from build123d import *

# Parameters (mm, degrees)
SKETCH1_W           = 50
SKETCH1_H           = 50
BOSS_EXTRUDE1_DEPTH = 10
LOFT1_START         = -25
LOFT1_DEPTH         = 50
SKETCH4_R           = 1.6
CUT_EXTRUDE1_DEPTH  = 4
SKETCH6_R           = 1.6
CUT_EXTRUDE2_DEPTH  = 4
FILLET1_R           = 10
CUT_EXTRUDE4_DEPTH  = 1


# Read off the part's stored shape, not the designer's step: Loft1
with BuildPart() as part:
    # Sketch1 → Boss-Extrude1 (new body)
    with BuildSketch(Plane(origin=(0, 0, 0), x_dir=(1, 0, 0), z_dir=(0, 1, 0))):
        Rectangle(SKETCH1_W, SKETCH1_H)
    extrude(amount=BOSS_EXTRUDE1_DEPTH)

    # Loft1 outline → Loft1 (add)
    with BuildSketch(Plane.XY.offset(LOFT1_START)):
        Polygon((25, 0), (-25, 0), (24.904867452, -2.178893569), align=None)
    extrude(amount=LOFT1_DEPTH)

    # Sketch4 → Cut-Extrude1 (cut)
    with BuildSketch(Plane(origin=(-0.047566274, -1.089446784, 0), x_dir=(0.9990482215818578, -0.043619387365336104, 0), z_dir=(-0.043619387365336104, -0.9990482215818578, 0))):
        with Locations((20, 20)):
            Circle(SKETCH4_R)
        with Locations((20, -20)):
            Circle(SKETCH4_R)
        with Locations((-20, -20)):
            Circle(SKETCH4_R)
        with Locations((-20, 20)):
            Circle(SKETCH4_R)
    extrude(amount=-CUT_EXTRUDE1_DEPTH, mode=Mode.SUBTRACT)

    # Sketch6 → Cut-Extrude2 (cut)
    with BuildSketch(Plane(origin=(0, 10, 0), x_dir=(1, 0, 0), z_dir=(0, 1, 0))):
        with Locations(Location((21, 21, 0), (0, 0, 270))):
            Circle(SKETCH6_R)
        with Locations(Location((21, -21, 0), (0, 0, 270))):
            Circle(SKETCH6_R)
        with Locations(Location((-21, -21, 0), (0, 0, 270))):
            Circle(SKETCH6_R)
        with Locations(Location((-21, 21, 0), (0, 0, 270))):
            Circle(SKETCH6_R)
    extrude(amount=-CUT_EXTRUDE2_DEPTH, mode=Mode.SUBTRACT)

    # Fillet1
    # the kernel refuses this fillet: 10 mm, written as the material it takes off along each edge
    with BuildSketch(Plane(origin=(25, 0, -25.545501942), x_dir=(0, 1, 0), z_dir=(0, 0, 1))) as fillet1_piece_1:
        with BuildLine():
            CenterArc((FILLET1_R * 0.0218200776863, FILLET1_R), FILLET1_R, 267.499999993, 2.500000007)
            Line((-FILLET1_R * 0.0217993098072, FILLET1_R * 0.00095177842374), (0, 0))
            Line((0, 0), (FILLET1_R * 0.0218200776863, 0))
        make_face()
    extrude(amount=51.091003884, mode=Mode.SUBTRACT)

    # Sketch8 → Cut-Extrude4 (cut)
    # profile 1 of 2: a face of its own
    with BuildSketch(Plane.XY.offset(25)):
        with BuildLine():
            Line((-2.597489017, 8.20661879), (-1.993908288, 8.207890825))
            Line((-1.993908288, 8.207890825), (-1.990092182, 6.164366186))
            add(Edge.make_bspline(
                [(-1.990092182, 6.164366186), (-1.990044981, 6.143161949), (-1.989954316, 6.102432362), (-1.98719006, 6.043693532), (-1.983535675, 5.989812448), (-1.978474748, 5.940590206), (-1.972213443, 5.896230054), (-1.964810654, 5.856420037), (-1.955356589, 5.821562302), (-1.941074869, 5.781805473), (-1.918545267, 5.737393222), (-1.88297912, 5.690959505), (-1.840900192, 5.649204853), (-1.791278495, 5.613903537), (-1.735063778, 5.584986173), (-1.672775576, 5.56486761), (-1.605162185, 5.552435164), (-1.558292927, 5.551231377), (-1.534067542, 5.550609174)],
                knots=[0, 0, 0, 0, 1.152644125, 2.214025477, 3.196161738, 4.088430453, 4.903432181, 5.631297626, 6.288373025, 6.86443571, 7.926317597, 8.979784177, 10.031167994, 11.137891127, 12.27708747, 13.454363037, 14.684232779, 16, 16, 16, 16], degree=3))
            add(Edge.make_bspline(
                [(-1.534067542, 5.550609174), (-1.508342778, 5.551344218), (-1.458392144, 5.552771477), (-1.38647613, 5.567260105), (-1.320175779, 5.590067607), (-1.260159607, 5.621972608), (-1.207784977, 5.661229411), (-1.163051106, 5.705642718), (-1.126756521, 5.754903538), (-1.104539344, 5.801287384), (-1.090919789, 5.843176805), (-1.082446638, 5.881122654), (-1.074798653, 5.925478097), (-1.068502962, 5.975979624), (-1.064302042, 6.033085663), (-1.061178272, 6.096494834), (-1.059289451, 6.166474936), (-1.059074503, 6.215246414), (-1.058962374, 6.240688301)],
                knots=[0, 0, 0, 0, 1.271674988, 2.469253807, 3.614054625, 4.731162594, 5.818153213, 6.841986676, 7.840949062, 8.831111795, 9.371942087, 10.018382253, 10.75320863, 11.599114249, 12.535801032, 13.586328523, 14.740896136, 16, 16, 16, 16], degree=3))
            Line((-1.058962374, 6.240688301), (-1.06277848, 8.20916286))
            Line((-1.06277848, 8.20916286), (-0.459197751, 8.210434896))
            Line((-0.459197751, 8.210434896), (-0.455381645, 6.327822716))
            add(Edge.make_bspline(
                [(-0.455381645, 6.327822716), (-0.455427497, 6.289659556), (-0.455515647, 6.21629181), (-0.458289071, 6.110918126), (-0.461814303, 6.014630937), (-0.467384408, 5.927444116), (-0.475128208, 5.849211971), (-0.483609602, 5.779962438), (-0.494254852, 5.719827409), (-0.511101496, 5.651616734), (-0.540202063, 5.573125016), (-0.584540214, 5.481851601), (-0.643443749, 5.393738081), (-0.711846857, 5.308083315), (-0.789095734, 5.22867752), (-0.873562656, 5.158654821), (-0.964207697, 5.099802482), (-1.061217352, 5.05236512), (-1.164968764, 5.015852552), (-1.276248979, 4.989816387), (-1.395852353, 4.974728231), (-1.478266961, 4.972397474), (-1.520711172, 4.971197115)],
                knots=[0, 0, 0, 0, 1.153606413, 2.21778028, 3.186276612, 4.066178262, 4.858206436, 5.562506921, 6.174709129, 6.703194428, 7.684393792, 8.699014322, 9.763766974, 10.880761115, 12.0092423, 13.106350137, 14.190711311, 15.268404456, 16.362982341, 17.508657393, 18.716937746, 20, 20, 20, 20], degree=3))
            add(Edge.make_bspline(
                [(-1.520711172, 4.971197115), (-1.548921319, 4.971725785), (-1.604368835, 4.972764896), (-1.686183271, 4.979779), (-1.765227448, 4.991850187), (-1.841591746, 5.008854994), (-1.914983671, 5.031425855), (-1.98589913, 5.05802141), (-2.054022722, 5.089780937), (-2.118688428, 5.126683391), (-2.179562073, 5.167512676), (-2.236618712, 5.210440833), (-2.289443467, 5.255799025), (-2.336824872, 5.304275742), (-2.38072026, 5.354640261), (-2.419200428, 5.408131493), (-2.453865888, 5.463682585), (-2.484516032, 5.522820121), (-2.511340089, 5.588612717), (-2.532761656, 5.663826937), (-2.552116951, 5.748901286), (-2.566727329, 5.844173393), (-2.578801096, 5.949614065), (-2.58762407, 6.065232271), (-2.592496247, 6.191248581), (-2.593270756, 6.278633173), (-2.593672911, 6.32400661)],
                knots=[0, 0, 0, 0, 1.02296857, 2.010661828, 2.975102012, 3.920728081, 4.844890381, 5.757306083, 6.665306112, 7.567395873, 8.454421116, 9.321634866, 10.155527794, 10.976419367, 11.777782189, 12.575893134, 13.363117526, 14.150529598, 14.988558697, 15.934809602, 16.983005217, 18.150875452, 19.427780756, 20.831133413, 22.354602744, 24, 24, 24, 24], degree=3))
            Line((-2.593672911, 6.32400661), (-2.597489017, 8.20661879))
        make_face()
    # profile 2 of 2: a face of its own
    with BuildSketch(Plane.XY.offset(25)):
        with BuildLine():
            Line((0.751773127, 7.391012504), (0.751773127, 7.133425365))
            add(Edge.make_bspline(
                [(0.751773127, 7.133425365), (0.778472329, 7.158935271), (0.83075507, 7.208889119), (0.91540949, 7.274289424), (1.003299732, 7.329052484), (1.094438334, 7.374170373), (1.188742293, 7.408966836), (1.286127124, 7.435040483), (1.386924841, 7.449591081), (1.455165046, 7.451662404), (1.489553576, 7.452706214)],
                knots=[0, 0, 0, 0, 1.07236104, 2.099912038, 3.101509264, 4.076695536, 5.049251982, 6.017409511, 7.000906107, 8, 8, 8, 8], degree=3))
            add(Edge.make_bspline(
                [(1.489553576, 7.452706214), (1.526924592, 7.451800756), (1.600743213, 7.450012213), (1.709259158, 7.433628514), (1.813580931, 7.40703223), (1.913508294, 7.369042139), (2.009538866, 7.32069025), (2.100531928, 7.260258837), (2.187555401, 7.189924161), (2.269207456, 7.10944842), (2.34355068, 7.020307883), (2.409944412, 6.92481222), (2.464182597, 6.822021375), (2.510876223, 6.7143822), (2.545388061, 6.599620476), (2.570855741, 6.479240849), (2.586463156, 6.352591682), (2.588293394, 6.266153935), (2.589228055, 6.222012103)],
                knots=[0, 0, 0, 0, 0.97285607, 1.921673578, 2.851140669, 3.772105152, 4.700636827, 5.645590137, 6.611463219, 7.611062552, 8.626324728, 9.631081099, 10.634121403, 11.648482193, 12.682506745, 13.749260973, 14.85059771, 16, 16, 16, 16], degree=3))
            add(Edge.make_bspline(
                [(2.589228055, 6.222012103), (2.588298537, 6.179349915), (2.586474919, 6.095651135), (2.570706926, 5.972853752), (2.545603057, 5.855183022), (2.509168603, 5.742953987), (2.462478649, 5.636026689), (2.405516744, 5.534470889), (2.338601572, 5.437871439), (2.261335844, 5.348453672), (2.177246838, 5.267258834), (2.089530639, 5.194426949), (1.996891996, 5.133719372), (1.900067324, 5.084592613), (1.799825884, 5.045403376), (1.695598692, 5.017296578), (1.58741629, 5.000400903), (1.513994179, 4.998170845), (1.476833223, 4.997042151)],
                knots=[0, 0, 0, 0, 1.112323361, 2.182262823, 3.223467608, 4.246437882, 5.254246404, 6.261812182, 7.278802008, 8.313998772, 9.338537047, 10.324801996, 11.283349242, 12.220607119, 13.15197435, 14.085554928, 15.031046561, 16, 16, 16, 16], degree=3))
            add(Edge.make_bspline(
                [(1.476833223, 4.997042151), (1.443713635, 4.997866298), (1.37847004, 4.999489817), (1.28239675, 5.013308287), (1.18972649, 5.035554908), (1.099816742, 5.066844085), (1.011800444, 5.108860697), (0.925752316, 5.163179132), (0.838187871, 5.226650427), (0.783321035, 5.276537488), (0.754953215, 5.302330613)],
                knots=[0, 0, 0, 0, 0.987385084, 1.945089202, 2.888259662, 3.826137757, 4.779238709, 5.78997447, 6.857349733, 8, 8, 8, 8], degree=3))
            Line((0.754953215, 5.302330613), (0.756861268, 4.201384099))
            Line((0.756861268, 4.201384099), (0.175541156, 4.200748081))
            Line((0.175541156, 4.200748081), (0.170453015, 7.390376486))
            Line((0.170453015, 7.390376486), (0.751773127, 7.391012504))
        make_face()
        with BuildLine():
            add(Edge.make_bspline(
                [(1.368710227, 6.911455212), (1.346213252, 6.910793906), (1.301889553, 6.909490995), (1.236800882, 6.900703018), (1.174825335, 6.884952495), (1.115281841, 6.865000801), (1.058891287, 6.838102927), (1.006158968, 6.804454728), (0.955302726, 6.766437156), (0.908795742, 6.721898104), (0.866041178, 6.673203682), (0.829171668, 6.620171725), (0.797662517, 6.563797157), (0.772116057, 6.503651781), (0.752619184, 6.439615962), (0.737765481, 6.372266556), (0.7295235, 6.301085467), (0.728674715, 6.252561314), (0.728240475, 6.227736262)],
                knots=[0, 0, 0, 0, 1.027737872, 2.024856463, 2.992617016, 3.945137832, 4.889499754, 5.838073507, 6.798830374, 7.785357117, 8.773878476, 9.754540506, 10.730023958, 11.719398922, 12.733354597, 13.783839577, 14.866207966, 16, 16, 16, 16], degree=3))
            add(Edge.make_bspline(
                [(0.728240475, 6.227736262), (0.728932743, 6.202275745), (0.730280627, 6.152702693), (0.738422537, 6.08005334), (0.75306485, 6.011292092), (0.773556922, 5.946234461), (0.798907779, 5.884714778), (0.830366781, 5.826871472), (0.867820106, 5.773025683), (0.91065126, 5.723370351), (0.95726968, 5.678357076), (1.007763484, 5.639224622), (1.06153695, 5.6068128), (1.1177563, 5.579922387), (1.176954499, 5.558646747), (1.239181745, 5.543528138), (1.30440737, 5.534333858), (1.348751423, 5.533585019), (1.371254297, 5.533205012)],
                knots=[0, 0, 0, 0, 1.150869826, 2.240808007, 3.29890037, 4.323262251, 5.319818076, 6.30175507, 7.2932304, 8.278527964, 9.261212744, 10.217617135, 11.159266914, 12.093623991, 13.030189547, 13.99700188, 14.983556707, 16, 16, 16, 16], degree=3))
            add(Edge.make_bspline(
                [(1.371254297, 5.533205012), (1.393128622, 5.533793245), (1.436452488, 5.534958287), (1.499904241, 5.544898072), (1.560968418, 5.559972722), (1.618912299, 5.581746332), (1.674296494, 5.609496131), (1.727218439, 5.643057943), (1.776798655, 5.683723983), (1.823930937, 5.729037604), (1.865777732, 5.77989361), (1.904183947, 5.833232179), (1.935119368, 5.891270601), (1.961360615, 5.951971312), (1.981219465, 6.016410897), (1.994773785, 6.083982305), (2.004336984, 6.154747505), (2.005017408, 6.203110383), (2.005363872, 6.227736262)],
                knots=[0, 0, 0, 0, 0.998586769, 1.977781659, 2.926627622, 3.867334799, 4.798423245, 5.752050313, 6.722974502, 7.722781292, 8.733270033, 9.727291971, 10.719614403, 11.730474272, 12.744298273, 13.79263617, 14.876033113, 16, 16, 16, 16], degree=3))
            add(Edge.make_bspline(
                [(2.005363872, 6.227736262), (2.004660421, 6.252347386), (2.003285885, 6.300437262), (1.995240688, 6.371000149), (1.980354194, 6.437720012), (1.960745423, 6.50128771), (1.935176776, 6.561395106), (1.903915874, 6.617963719), (1.867459395, 6.6715612), (1.824828199, 6.720411759), (1.778956571, 6.765724093), (1.728833044, 6.804678965), (1.676093164, 6.83793361), (1.620131268, 6.864855463), (1.561466804, 6.885779245), (1.499970245, 6.901242858), (1.435343762, 6.910334609), (1.391212006, 6.911076791), (1.368710227, 6.911455212)],
                knots=[0, 0, 0, 0, 1.128965526, 2.20598662, 3.251153905, 4.259863426, 5.253177665, 6.241051661, 7.220081141, 8.219894056, 9.210062323, 10.172878603, 11.125229178, 12.064585276, 13.014948265, 13.977126056, 14.968582519, 16, 16, 16, 16], degree=3))
        make_face(mode=Mode.SUBTRACT)
    extrude(amount=-CUT_EXTRUDE4_DEPTH, mode=Mode.SUBTRACT)


solid = part.part
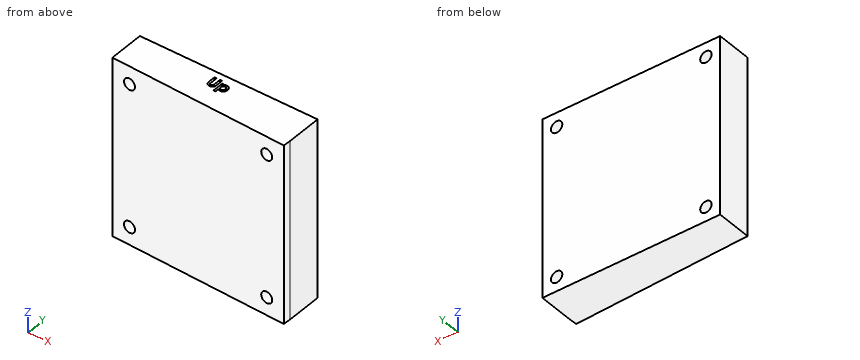
The model under review builds one solid part; all positions refer to its coordinate system, in mm. Give positions to 0.01 mm unless a question says otherwise; leave off trailing zeros. Loops run counter-clockwise (first coordinate to the right, second up) from the corner with the lowest first, then second, coordinate; pieces in that order, holes last. Notation, with made-up numbers: (-31.5, 57.5) -> (-23.5, 57.5) arc R10 ccw to (-23.5, 68.5) -> close; hole circle Ø8 at (76.5, 26.5). An arc over 180 degrees is marked (long way). Answer as a JSON object with one key per item and string values. Group by question number.
Q1. Take a section at A-A (z = 0). Write out the cut boundary in (x, y).
Q2. Take a section at B-B (x = -17). Write out the cut boundary in (y, z).
Q3. Take a section at D-D (x = 14). Write out the cut boundary in (y, z).
Q4. Take a section at C-C (z = 21). Write out the cut boundary in (x, y).
Q5. Wall thickness on line 1 along X through (y, z) = (8.2, 21); line 2 along Z through (x, y) = (19, -0.75); line 3 along Y through (x, z) = (10, 14): over which ranges is each line inside the solid? List them lowest first.
Q6. Insertion check: pin 1 (1.9 mm diameter, centred on x = -21, z = -21, fed in from +Y); pin 2 (4 mm diameter, centred on x = 19.5, z = -2.5, fed in from -Y); pin 3 (1.5 mm diameter, centred on x = -15, z = -10, fed in from -Y). Each pin has a flat end and moves straight along its axis. Give the tip position at first contact, or say it passes through.
Answer below:
{
 "1": {"outline": "(-25, 0) -> (24.9, -2.18) -> (24.99, -0.22) arc R10 ccw to (25, 0.22) -> (25, 10) -> (-25, 10) -> close"},
 "2": {"outline": "(-0.35, -25) -> (10, -25) -> (10, 25) -> (-0.35, 25) -> close"},
 "3": {"outline": "(-1.7, -25) -> (10, -25) -> (10, 25) -> (-1.7, 25) -> close"},
 "4": {"outline": "(-25, 0) -> (-21.28, -0.16) -> (-21.1, 3.83) -> (-18.61, 3.72) -> (-18.78, -0.27) -> (18.69, -1.91) -> (18.86, 2.09) -> (21.36, 1.98) -> (21.18, -2.02) -> (24.9, -2.18) -> (24.99, -0.22) arc R10 ccw to (25, 0.22) -> (25, 10) -> (22.6, 10) -> (22.6, 6) -> (19.4, 6) -> (19.4, 10) -> (-19.4, 10) -> (-19.4, 6) -> (-22.6, 6) -> (-22.6, 10) -> (-25, 10) -> close"},
 "5": {"line 1": "x = -25 to -22.6, -19.4 to 19.4, 22.6 to 25", "line 2": "z = -25 to -21.26, -18.74 to 18.74, 21.26 to 25", "line 3": "y = -1.53 to 10"},
 "6": {"pin 1": "stops at y = 6", "pin 2": "stops at y = -2.03", "pin 3": "stops at y = -0.47"}
}
